Can you work these out from the drawing? Everything is in mm from the part's minimum corner. Round coordinates to 2 decimals unless told otherwise and drop trailing zeros. Loops run counter-clockwise (first coordinate to the right, second up) from the corner with the lowest first, then second, coordinate; pieces in that order, holes last. Notation, with made-up numbers: M -22,33 L 34,33 A22 cw 34,55 Z; hole C 49.25,64.25 d7. An arc over 180 degrees is marked long. Return JSON: item names as keys, results as strings. Group by question number.
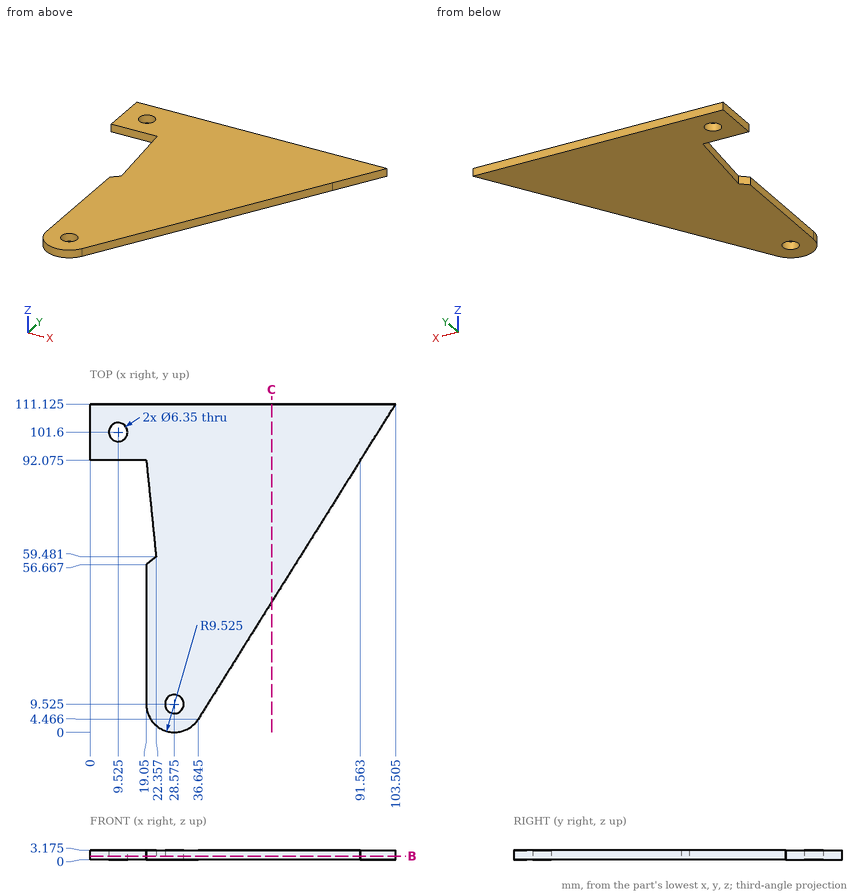
1. I'm going to push flat-ended pins straight in: pin 1 Ø1.5 at (y, z) = (12, 1) entering from +X; pin 2 Ø1 at (y, z) = (62.5, 3) entering from -X; pin 3 Ø1.6 at (y, z) = (34, 1.5) entering from -X. Where does each tip first touch, or does it pass through?
2. I need wall thicknesses on probe 1 along Y at (x, z) = (11.5, 0.65) (1 decimal); probe 2 along Y at (x, z) = (15, 0.5) (1 decimal); probe 3 along Y at (x, z) = (39, 2.55) (1 decimal). Which ranges of each line are inside material? Lowest first, please.
3. If we section it at B-B, the plane z = 1.2: Give the number of separate pieces and of enclosed holes in the cut face, then the cut area to 3 significant figures.
4. If we section it at C-C, the plane x = 61.5: Please give me the cut outline in (y, z) (1 decimal), then the cut area to 3 significant figures.
Geometry results:
{
 "1": {"pin 1": "x = 41.84", "pin 2": "x = 22", "pin 3": "x = 19.05"},
 "2": {"probe 1": "92.1 to 99.1, 104.1 to 111.1", "probe 2": "92.1 to 111.1", "probe 3": "8.2 to 111.1"},
 "3": {"separate pieces": "1", "enclosed holes": "2", "area": "5,730 mm^2"},
 "4": {"outline": "M 44.1,0 L 111.1,0 L 111.1,3.2 L 44.1,3.2 Z", "area": "213 mm^2"}
}
